Geometry: final body of the model. Coordinates: model frame, mm. Face numbers are marked on the shaded views. A direction names the side the tool comes from. Round coordinates to 2 decimals unless told otherwise and drop trailing zeros. Loops run counter-clockwise (first coordinate to the right, second up) from the corner with the lowest first, then second, coordinate; pieces in that order, holes last. Notation, with made-up numbers: (39, 3) - (94, 3) arc R24 cw to (94, 37) - close; hole circle Ø5 at (76.5, -6). An arc over 180 degrees is marked (long way). Return JSON: item names as keys, results as strings. Group by question number.
1. Draft query along X for the marked faces 1, 2, 3 and 4. Return one class per face: +X half, -X half, draft (parallel to the pull), parting line (faces both ways), or undercut.
2. First-contact query: pin 1 Ø2 at (x, y) = (-203, -28) entering from -Z; pin 2 Ø1.5 at (x, y) = (262, -225.5) entering from +Z; pin 3 Ø11.5 at (x, y) = (-240, -294.5) entering from -Z. Flat tips, straight axial feed; report the tip coordinate or a pass-through.
3. Section A-A on z = 103. Return loops of the section in (x, y).
4. Set-up query: the marked faces 5, 6 and 7. Return all of +Z, -Z, +X, -X, +Y, -Y with unobstructed straight access to the full face (end or side cutting, diameter ignored); none if empty.
5. Section C-C on x = 369. Return loops of the section in (y, z), and give its area (3 significant figures).
6. Material intervals for probe 1 along X at (y, z) = (-113, -35); probe 2 along X at (y, z) = (-244.5, 87.5); probe 3 along Y at (x, z) = (-229.5, -27), sorted ascending.
7. Section D-D on z = -93.5. Return loops of the section in (x, y).
8. Section B-B on y = -51. Return loops of the section in (x, z), and give its area (3 significant figures).
from build123d import *

# Parameters (mm, degrees)
F0_W      = 914.4
F0_H      = 381
F1_DEPTH  = 50.8
F2_R      = 127
F3_DEPTH  = 50.8
F4_R      = 127
F5_DEPTH  = 50.8
F6_W      = 101.6
F6_H      = 254
F7_DEPTH  = 38.1
F8_W      = 101.6
F8_H      = 76.2
F9_DEPTH  = 76.2
F10_W     = 101.6
F10_H     = 76.2
F11_DEPTH = 63.5


with BuildPart() as f1:
    # F0 (on Top) → F1 (new body)
    with BuildSketch(Plane.XY):
        with Locations((1.296762, -93.692474)):
            Rectangle(F0_W, F0_H)
    extrude(amount=F1_DEPTH)

    # F2 (on face) → F3 (join)
    with BuildSketch(Plane.YZ.offset(458.496762)):
        with Locations((-93.692474, 0)):
            Circle(F2_R)
    extrude(amount=F3_DEPTH)

    # F4 (on face) → F5 (join)
    with BuildSketch(Plane(origin=(-455.903238, 0, 0), x_dir=(0, -1, 0), z_dir=(-1, 0, 0))):
        with Locations((93.692474, 0)):
            Circle(F4_R)
    extrude(amount=F5_DEPTH)

    # F6 (on face) → F7 (join)
    with BuildSketch(Plane.XZ.offset(284.192474)):
        with Locations((-227.303238, 9.129721)):
            Rectangle(F6_W, F6_H)
        with Locations((229.896762, -1.581132)):
            Rectangle(F6_W, F6_H)
    extrude(amount=F7_DEPTH)

    # F8 (on face) → F9 (join)
    with BuildSketch(Plane.XY.offset(50.8)):
        with Locations((-227.303238, -246.092474)):
            Rectangle(F8_W, F8_H)
    extrude(amount=F9_DEPTH)

    # F10 (on face) → F11 (join)
    with BuildSketch(Plane.XY.offset(50.8)):
        with Locations((229.896762, -246.092474)):
            Rectangle(F10_W, F10_H)
    extrude(amount=F11_DEPTH)


solid = f1.part
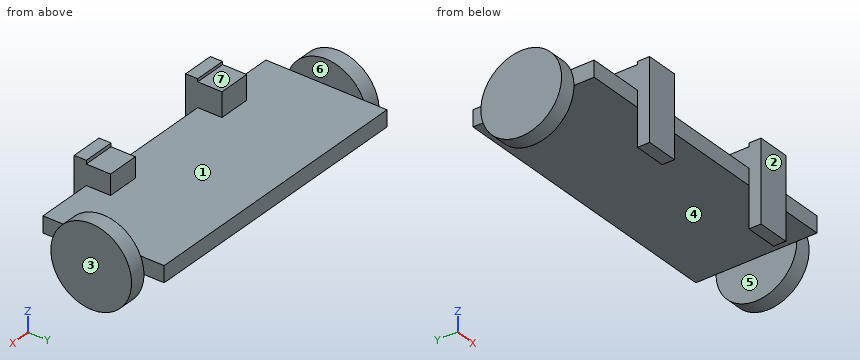
Taken from the geometry:
{
 "1": {"face 1": "undercut", "face 2": "draft", "face 3": "+X half", "face 4": "undercut"},
 "2": {"pin 1": "z = 0", "pin 2": "z = 114.3", "pin 3": "z = -117.87"},
 "3": {"outline": "(-506.7, -167.99) - (-455.9, -167.99) - (-455.9, -19.4) - (-506.7, -19.4) - close; (-278.1, -322.29) - (-176.5, -322.29) - (-176.5, -207.99) - (-278.1, -207.99) - close; (179.1, -322.29) - (280.7, -322.29) - (280.7, -207.99) - (179.1, -207.99) - close; (458.5, -167.99) - (509.3, -167.99) - (509.3, -19.4) - (458.5, -19.4) - close"},
 "4": {"face 5": "-Z, +Y, -Y", "face 6": "+Z, +Y, -Y", "face 7": "+Z, +X, -X, +Y"},
 "5": {"outline": "(-284.19, 0) - (96.81, 0) - (96.81, 50.8) - (-284.19, 50.8) - close", "area": "19,400 mm2"},
 "6": {"probe 1": "-506.7 to -455.9, 458.5 to 509.3", "probe 2": "-278.1 to -176.5, 179.1 to 280.7", "probe 3": "-322.29 to -284.19"},
 "7": {"outline": "(-506.7, -179.64) - (-455.9, -179.64) - (-455.9, -7.75) - (-506.7, -7.75) - close; (-278.1, -322.29) - (-176.5, -322.29) - (-176.5, -284.19) - (-278.1, -284.19) - close; (179.1, -322.29) - (280.7, -322.29) - (280.7, -284.19) - (179.1, -284.19) - close; (458.5, -179.64) - (509.3, -179.64) - (509.3, -7.75) - (458.5, -7.75) - close"},
 "8": {"outline": "(-506.7, -119.61) - (-455.9, -119.61) - (-455.9, 0) - (458.5, 0) - (458.5, -119.61) - (509.3, -119.61) - (509.3, 119.61) - (458.5, 119.61) - (458.5, 50.8) - (-455.9, 50.8) - (-455.9, 119.61) - (-506.7, 119.61) - close", "area": "70,800 mm2"}
}
